Work out the finished part from the listing and answer in its coordinate system (mm). A direction names the side the tool comes from. Coordinates: 2 decimals unless noted, no trailing zeros. Order: outer loops, then holes, each group sorted by start corner. A loop starts at its lowest first (then second) coordinate and runs counter-clockwise, first axis right, second up.
1. The part is cut by section B-B, the plane y = 35. Give the vertices of the cut face in (x, z).
2. Flat-ended cylindrical pins translate along their axes: pin 1 Ø3 at (y, z) = (55.5, 3.5) entering from -X; pin 2 Ø1.9 at (y, z) = (24, 2.5) entering from +X; pin 3 Ø1.9 at (y, z) = (34.5, 3.5) entering from -X. Find the tip coordinate at first contact, or state that the pin passes through.
3. Find the intervals of material crossed by probe 1 along Y at (x, z) = (6.5, 5.75); probe 2 along Y at (x, z) = (-34, 2); probe 3 along Y at (x, z) = (16, 2), in increasing order.
4. A tool of negligible diameter and unlimited length cuts with its end or side. For faces 4 (the flat face through (5, 53.181, 3)), 5 (the flat face through (-27.987, 33, 3)), 6 (the cylindrical face through (-6.83, 60.8, 3.13)), from which of +Z, -Z, +X, -X, +Y, -Y can it reach the whole face along a straight path? Write none if from no direction.
5. Determine the mould class of faces 1 (the cylindrical face through (-40.17, 67.17, 3.22)), 2 (the flat face through (-41.618, 6, 3)), 3 (the cylindrical face through (20.434, 54.709, 3.219)) for opening direction Y: +Y half, -Y half, draft (parallel to the pull), parting line (faces both ways), or undercut.
6. The part is cut by section C-C, the plane z = 4.5. Count the separate pieces of the cut face and the enclosed holes in it, then the cut area to 3 significant figures.
7. The part is cut by section A-A, the plane x = 14. Give the vertices of the cut face in (y, z).
```python
from build123d import *

# Parameters (mm, degrees)
F0_R     = 1.5875
F0_W     = 21.5011
F0_H     = 40.48125
F1_DEPTH = 6.35
F2_R     = 5.08


with BuildPart() as f1:
    # F0 (on Top) → F1 (new body)
    with BuildSketch(Plane.XY):
        Polygon((-41.617566, 53.18125), (-27.986656, 53.18125), (-6.485556, 53.18125), (21.882434, 53.18125), (21.882434, 68.69938), (-41.617566, 68.69938), align=None)
        with Locations((-27.986656, 62.34938)):
            Circle(F0_R, mode=Mode.SUBTRACT)
        with Locations((-6.485556, 62.34938)):
            Circle(F0_R, mode=Mode.SUBTRACT)
        with Locations((-17.236106, 32.940625)):
            Rectangle(F0_W, F0_H)
        Polygon((-41.617566, 12.7), (-41.617566, 0), (21.882434, 0), (21.882434, 12.7), (-6.485556, 12.7), (-27.986656, 12.7), align=None)
        with BuildLine():
            ThreePointArc((-32.886316, 7.9375), (-33.349189, 6.817068), (-34.467883, 6.350011))
            ThreePointArc((-34.467883, 6.350011), (-34.47085, 6.350003), (-34.473816, 6.35))
            ThreePointArc((-34.473816, 6.35), (-35.596348, 9.060032), (-32.886316, 7.9375))
        make_face(mode=Mode.SUBTRACT)
        with BuildLine():
            ThreePointArc((13.151184, 6.35), (14.738684, 7.9375), (16.326184, 6.35))
            ThreePointArc((16.326184, 6.35), (14.738684, 4.7625), (13.151184, 6.35))
        make_face(mode=Mode.SUBTRACT)
    extrude(amount=F1_DEPTH)

    # F2
    f2_edges = [f1.edges().sort_by_distance(p)[0] for p in [
        (21.882434, 0, 3.175),
        (21.882434, 12.7, 3.175),
        (-41.617566, 0, 3.175),
        (-41.617566, 12.7, 3.175),
        (21.882434, 53.18125, 3.175),
        (21.882434, 68.69938, 3.175),
        (-41.617566, 53.18125, 3.175),
        (-41.617566, 68.69938, 3.175),
    ]]
    fillet(f2_edges, radius=F2_R)


solid = f1.part
```
Geometry says:
1. outline: (-27.99, 0) - (-6.49, 0) - (-6.49, 6.35) - (-27.99, 6.35) - close
2. pin 1: stops at x = -41.46
2. pin 2: stops at x = -6.49
2. pin 3: stops at x = -27.99
3. probe 1: y = 0 to 12.7, 53.18 to 68.7
3. probe 2: y = 0 to 6.42, 9.45 to 12.7, 53.18 to 68.7
3. probe 3: y = 0 to 5.39, 7.31 to 12.7, 53.18 to 68.7
4. face 4: +Z, -Z, +X
4. face 5: +Z, -Z, -X
4. face 6: +Z, -Z
5. face 1: +Y half
5. face 2: draft
5. face 3: undercut
6. separate pieces: 1
6. enclosed holes: 4
6. area: 2,590 mm2
7. outline: (0, 0) - (4.94, 0) - (4.94, 6.35) - (0, 6.35) - close; (7.76, 0) - (12.7, 0) - (12.7, 6.35) - (7.76, 6.35) - close; (53.18, 0) - (68.7, 0) - (68.7, 6.35) - (53.18, 6.35) - close
